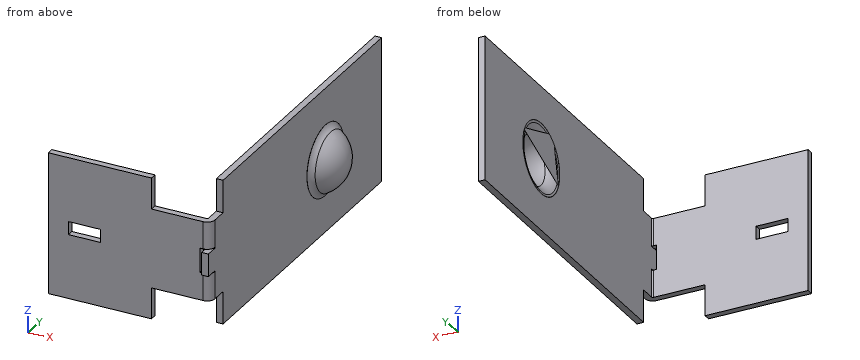
```python
from build123d import *
from build123d.topology import SkipClean

# Parameters (mm, degrees)
Y_KSEKLIK_EKSTR_ZYON1_DEPTH = 3.24
IZIM2_W                     = 1.429951724
IZIM2_H                     = 0.588312172
KES_EKSTR_ZYON1_DEPTH       = 1.04186858
KES_EKSTR_ZYON2_DEPTH       = 0.5
Y_KSEKLIK_EKSTR_ZYON2_DEPTH = 0.3
IZIM7_R                     = 1.580293975
KES_EKSTR_ZYON3_DEPTH       = 0.3


with BuildPart() as part:
    # izim1 → Y_kseklik-Ekstr_zyon1 (new, symmetric)
    with BuildSketch(Plane.XY):
        with BuildLine():
            Line((-0.3, 0.35), (-0.3, 14.676))
            Line((-0.3, 14.676), (0, 14.676))
            Line((0, 14.676), (0, 0.35))
            ThreePointArc((0, 0.35), (-0.102512627, 0.102512627), (-0.35, 0))
            Line((-0.35, 0), (-7.3, 0))
            Line((-7.3, 0), (-7.3, 0.3))
            Line((-7.3, 0.3), (-0.35, 0.3))
            ThreePointArc((-0.35, 0.3), (-0.314644661, 0.314644661), (-0.3, 0.35))
        make_face()
    extrude(amount=Y_KSEKLIK_EKSTR_ZYON1_DEPTH, both=True)

    # izim2 → Kes-Ekstr_zyon1 (cut)
    with BuildSketch(Plane(origin=(0, 0, 0), x_dir=(1, 0, 0), z_dir=(0, 1, 0))):
        Polygon((0, -4), (0, -1.778), (-2.671699332, -1.778), (-2.671699332, -3.175), (-7.3, -3.175), (-7.3, 3.175), (-2.671699332, 3.175), (-2.671699332, 1.778), (0, 1.778), (0, 4), (-8, 4), (-8, -4), align=None)
        with Locations((-5.68100521, 0)):
            Rectangle(IZIM2_W, IZIM2_H)
    extrude(amount=KES_EKSTR_ZYON1_DEPTH, mode=Mode.SUBTRACT)

    # izim4 → Kes-Ekstr_zyon2 (cut)
    with BuildSketch(Plane(origin=(0, 0, 0), x_dir=(0, 0, -1), z_dir=(1, 0, 0))):
        with BuildLine():
            Line((-0.55, -0.15), (0.55, -0.15))
            Line((0.55, -0.15), (0.55, 0.33))
            ThreePointArc((0.55, 0.33), (0.544142136, 0.344142136), (0.53, 0.35))
            Line((0.53, 0.35), (-0.53, 0.35))
            ThreePointArc((-0.53, 0.35), (-0.544142136, 0.344142136), (-0.55, 0.33))
            Line((-0.55, 0.33), (-0.55, -0.15))
        make_face()
    extrude(amount=-KES_EKSTR_ZYON2_DEPTH, mode=Mode.SUBTRACT)

    # izim5 → Y_kseklik-Ekstr_zyon2 (add)
    with BuildSketch(Plane(origin=(0, 0, 0), x_dir=(0, 0, -1), z_dir=(1, 0, 0))):
        with BuildLine():
            Line((-0.51, -0.22), (0.51, -0.22))
            Line((0.51, -0.22), (0.51, 0.33))
            ThreePointArc((0.51, 0.33), (0.515857864, 0.344142136), (0.53, 0.35))
            Line((0.53, 0.35), (-0.53, 0.35))
            ThreePointArc((-0.53, 0.35), (-0.515857864, 0.344142136), (-0.51, 0.33))
            Line((-0.51, 0.33), (-0.51, -0.22))
        make_face()
    extrude(amount=-Y_KSEKLIK_EKSTR_ZYON2_DEPTH)

    # izim7 → Kes-Ekstr_zyon3 (cut)
    with BuildSketch(Plane(origin=(0, 0, 0), x_dir=(0, 0, -1), z_dir=(1, 0, 0))):
        with Locations((0, 9.847993975)):
            Circle(IZIM7_R)
    extrude(amount=-KES_EKSTR_ZYON3_DEPTH, mode=Mode.SUBTRACT)

    # izim6 → D_nd_r1 (revolve)
    with SkipClean():  # the faces are left unmerged after this step: merging them gives an invalid solid
        with BuildSketch(Plane.XY, mode=Mode.PRIVATE) as d_nd_r1_sk:
            with BuildLine():
                Line((0.716, 9.84078795), (1.0208, 9.84078795))
                ThreePointArc((1.0208, 9.84078795), (0.809273292, 10.612424612), (0.233830611, 11.168331447))
                ThreePointArc((0.233830611, 11.168331447), (0.096469293, 11.278181577), (0.0048, 11.42828795))
                Line((0.0048, 11.42828795), (-0.3, 11.42828795))
                ThreePointArc((-0.3, 11.42828795), (-0.294678979, 11.371583617), (-0.278901698, 11.316859108))
                ThreePointArc((-0.278901698, 11.316859108), (-0.132230828, 11.076688911), (0.08754728, 10.900928704))
                ThreePointArc((0.08754728, 10.900928704), (0.547080424, 10.456996364), (0.716, 9.84078795))
            make_face()
        revolve(d_nd_r1_sk.sketch.rotate(Axis((-0.492405336, 9.84078795, 0), (1, 0, 0)), 90), axis=Axis((-0.492405336, 9.84078795, 0), (1, 0, 0)))


solid = part.part
```
Verification items for the finished model (mm, model axes). Round coordinates to 2 decimals unless told otherwise and drop trailing zeros. Write each loop counter-clockwise with the first axis right and the second up, starting at its lowest first coordinate (ties: lowest second). Pieces come first, ordered by that corner, then holes. Notation, with made-up numbers: (64.25, 34) -> (79.25, 34) arc R18 cw to (79.25, 39) -> close; hole circle Ø10 at (-31.75, 18.25). An arc over 180 degrees is marked (long way). Write each question's results on one line, items separated by ' | '.
Q1. Go/stop test with flat-tipped pins: pin 1 Ø1.1 at (x, y) = (-1.5, 0.5) entering from +Z; pin 2 Ø3 at (y, z) = (4, -0.5) entering from +X; pin 3 Ø1 at (y, z) = (6.5, 2.5) entering from -X. Record where each tip stops, or that it passes through.
Derived:
pin 1: stops at z = 1.78 | pin 2: stops at x = 0 | pin 3: stops at x = -0.3
Q2. Thickness scan on probe 1 along X at (y, z) = (7, 2); probe 2 along Y at (x, z) = (-4, 1.5); probe 3 along X at (y, z) = (8.75, -0.25). Record the ranges inside material, lowest first.
Derived:
probe 1: x = -0.3 to 0 | probe 2: y = 0 to 0.3 | probe 3: x = 0 to 0.53
Q3. Sectioned sample at B-B, the plane x = -3.5. Record the boundary of the cut face in (y, z) (3 decimals), and give its area (4 significant figures).
Derived:
outline: (0, -3.175) -> (0.3, -3.175) -> (0.3, 3.175) -> (0, 3.175) -> close | area: 1.905 mm²
Q4. Sectioned sample at A-A, the plane y = 5.5. Record the boundary of the cut face in (x, z), and give its area (3 significant figures).
Derived:
outline: (-0.3, -3.24) -> (0, -3.24) -> (0, 3.24) -> (-0.3, 3.24) -> close | area: 1.94 mm²
